Work out the finished part from the listing and answer in its coordinate system (mm). Face numbers are marked on the shaded views. A direction names the side the tool comes from. Round coordinates to 2 decimals unless told otherwise and drop trailing zeros. Order: outer loops, then holes, each group sorted by start corner. A loop starts at its lowest first (then second) coordinate and runs counter-clockwise, first axis right, second up. Notation, with made-up numbers: (-33, 84) - (-2, 84) arc R25 ccw to (-2, 121) - close; hole circle Ø4 at (-13.75, 0.25). An arc over 180 degrees is marked (long way). Answer in a Markdown table with one row per item.
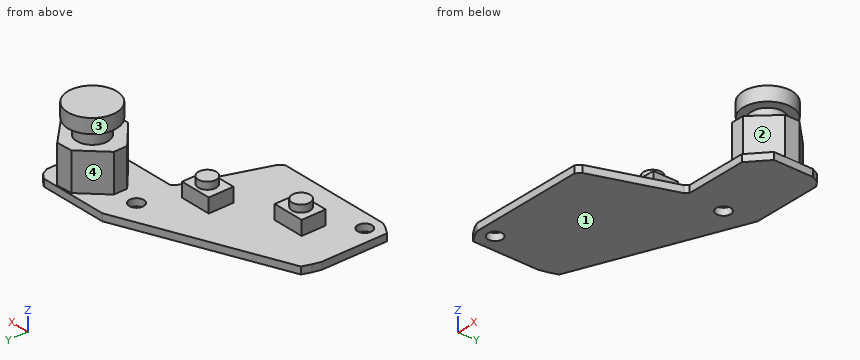
from build123d import *

# Parameters (mm, degrees)
SKETCH031_R     = 1.011832
PAD027_DEPTH    = 1
SKETCH032_W     = 4.41637
SKETCH032_H     = 3.379875
SKETCH032_W_2   = 4.371405
SKETCH032_H_2   = 3.470269
PAD028_DEPTH    = 3
PAD029_DEPTH    = 2.3
SKETCH034_R     = 2.204503
PAD030_DEPTH    = 4
SKETCH035_R     = 3.424311
PAD031_DEPTH    = 2
SKETCH036_W     = 18.521845
SKETCH036_H     = 12.987429
SKETCH036_R     = 1.2680878078
POCKET007_DEPTH = 1


with BuildPart() as part:
    # Sketch031 → Pad027 (new body)
    with BuildSketch(Plane.XY):
        Polygon((-15.824113, 0.702012), (-16.104103, -0.397312), (-16.104103, -9.622469), (-14.917328, -10.371682), (-14.188362, -10.695666), (1.802157, -10.695666), (2.429877, -10.099644), (6.254575, 0.878554), (6.659555, 1.344282), (15.224892, 1.344282), (17.820574, 3.648021), (17.820574, 9.166112), (17.347485, 10.117816), (16.497025, 10.725287), (6.898985, 10.725287), (-15.4012, 1.910333), align=None)
        with Locations((-13.754142, -8.512947)):
            Circle(SKETCH031_R, mode=Mode.SUBTRACT)
        with Locations((6.163737, 6.548235)):
            Circle(SKETCH031_R, mode=Mode.SUBTRACT)
    extrude(amount=PAD027_DEPTH)

    # Sketch032 (on Face20 of Pad027) → Pad028 (join)
    with BuildSketch(Plane.XY.offset(1)):
        with Locations((-8.389468, -4.0162585)):
            Rectangle(SKETCH032_W, SKETCH032_H)
        with Locations((1.6375455, 0.4002435)):
            Rectangle(SKETCH032_W_2, SKETCH032_H_2)
        Polygon((9.090246, 7.237029), (12.289592, 10.476871), (14.496734, 10.557867), (17.696077, 7.338274), (17.696077, 5.333621), (14.57773, 2.073529), (12.735069, 2.073529), (9.090246, 5.35387), align=None)
    extrude(amount=PAD028_DEPTH)

    # Pad028 Face39 → Pad029 (add)
    with BuildSketch(Plane(origin=(13.4460203648, 6.3372919202, 4), x_dir=(0, 1, 0), z_dir=(0, 0, 1))):
        Polygon((4.1395790798, 1.1564283648), (0.8997370798, 4.3557743648), (-0.9834219202, 4.3557743648), (-4.2637629202, 0.7109513648), (-4.2637629202, -1.1317096352), (-1.0036709202, -4.2500566352), (1.0009820798, -4.2500566352), (4.2205750798, -1.0507136352), align=None)
    extrude(amount=PAD029_DEPTH)

    # Sketch034 (on Face47 of Pad029) → Pad030 (join)
    with BuildSketch(Plane.XY.offset(6.3)):
        with Locations((13.367406, 6.580182)):
            Circle(SKETCH034_R)
    extrude(amount=PAD030_DEPTH)

    # Sketch035 (on Face49 of Pad030) → Pad031 (join)
    with BuildSketch(Plane.XY.offset(10.3)):
        with Locations((13.437232, 6.533877)):
            Circle(SKETCH035_R)
    extrude(amount=-PAD031_DEPTH)

    # Sketch036 (on Face38 of Pad031) → Pocket007 (cut)
    with BuildSketch(Plane.XY.offset(4)):
        with Locations((-4.0809855, -1.9936815)):
            Rectangle(SKETCH036_W, SKETCH036_H)
        with Locations((1.724279, 0.373466)):
            Circle(SKETCH036_R, mode=Mode.SUBTRACT)
        with Locations((-8.450182, -4.094334)):
            Circle(SKETCH036_R, mode=Mode.SUBTRACT)
    extrude(amount=-POCKET007_DEPTH, mode=Mode.SUBTRACT)


solid = part.part
1) Find section C-C, the plane x = -9. Give the vertices of the cut face in (y, z).
Filled in:
| item | result |
|---|---|
| outline | (-10.7, 0) - (4.44, 0) - (4.44, 1) - (-2.33, 1) - (-2.33, 3) - (-2.95, 3) - (-2.95, 4) - (-5.24, 4) - (-5.24, 3) - (-5.71, 3) - (-5.71, 1) - (-10.7, 1) - close |
2) Find section D-D, the plane z = 3.5. Give the vertices of the cut face in (x, y).
Filled in:
| item | result |
|---|---|
| outline | circle Ø2.54 at (-8.45, -4.09); circle Ø2.54 at (1.72, 0.37); (9.09, 5.35) - (12.74, 2.07) - (14.58, 2.07) - (17.7, 5.33) - (17.7, 7.34) - (14.5, 10.56) - (12.29, 10.48) - (9.09, 7.24) - close |
3) Find section A-A, the plane z = 2. Give the vertices of the cut face in (x, y).
Filled in:
| item | result |
|---|---|
| outline | (-10.6, -5.71) - (-6.18, -5.71) - (-6.18, -2.33) - (-10.6, -2.33) - close; (-0.55, -1.33) - (3.82, -1.33) - (3.82, 2.14) - (-0.55, 2.14) - close; (9.09, 5.35) - (12.74, 2.07) - (14.58, 2.07) - (17.7, 5.33) - (17.7, 7.34) - (14.5, 10.56) - (12.29, 10.48) - (9.09, 7.24) - close |
4) Find section B-B, the plane y = -4.75. Give the vertices of the cut face in (x, z), then the cut area to 3 significant figures.
Filled in:
| item | result |
|---|---|
| outline | (-16.1, 0) - (4.29, 0) - (4.29, 1) - (-6.18, 1) - (-6.18, 3) - (-7.36, 3) - (-7.36, 4) - (-9.54, 4) - (-9.54, 3) - (-10.6, 3) - (-10.6, 1) - (-16.1, 1) - close |
| area | 31.4 mm^2 |
5) Each of these flat-tipped pins is pushed along its axis until it touches: pin 1 (2 mm diameter, centred on x = 2, y = 0, fed in from +Z); pin 2 (0.6 mm diameter, centred on x = 0.5, z = 1.5, fed in from -Y); pin 3 (1 mm diameter, centred on x = -8.5, z = 2, fed in from -Y); pin 4 (1.8 mm diameter, centred on x = -13.75, y = -8.51, fed in from -Z). Where does it stop, or does it pass through?
Filled in:
| item | result |
|---|---|
| pin 1 | stops at z = 4 |
| pin 2 | stops at y = -1.33 |
| pin 3 | stops at y = -5.71 |
| pin 4 | passes through |
6) Which of the six approach directions +Z, -Z, +X, -X, +Y, -Y give full straight-line access (tool end or side, diameter ignored) to the marked faces 1, 2, 3 and 4?
Filled in:
| item | result |
|---|---|
| face 1 | -Z, +X, -X, +Y, -Y |
| face 2 | +Z, +X, -Y |
| face 3 | +Z |
| face 4 | +Z, -X, +Y |
7) Find the intervals of material crossed by probe 1 along Z at (x, y) = (0.5, 5.75); probe 2 along X at (y, z) = (6, 4); probe 3 along X at (y, z) = (-0.75, 2.5), in increasing order. Write a range as from..to.
Filled in:
| item | result |
|---|---|
| probe 1 | z = 0..1 |
| probe 2 | x = 9.09..17.7 |
| probe 3 | x = -0.55..3.82 |
